```python
from build123d import *

# Parameters (mm, degrees)
BOSS_EXTRUDE1_DEPTH = 5.5
BOSS_EXTRUDE2_DEPTH = 7.5
SKETCH4_R           = 2.5
CUT_EXTRUDE1_DEPTH  = 41.401113846
FILLET1_R           = 2
SKETCH5_R           = 2
FILLET2_RADIUS      = 5.5
FILLET2_LENGTH      = 18
FILLET3_RADIUS      = 5.5
FILLET3_LENGTH      = 18


with BuildPart() as part:
    # Sketch1 → Boss-Extrude1 (new, symmetric)
    with BuildSketch(Plane.XY):
        with BuildLine():
            Line((19, 0), (30, 0))
            Line((30, 0), (30, -18))
            Line((30, -18), (18.761663039, -18))
            ThreePointArc((18.761663039, -18), (0, -26), (-18.761663039, -18))
            Line((-18.761663039, -18), (-30, -18))
            Line((-30, -18), (-30, 0))
            Line((-30, 0), (-19, 0))
            ThreePointArc((-19, 0), (0, -19), (19, 0))
        make_face()
    extrude(amount=BOSS_EXTRUDE1_DEPTH, both=True)

    # Sketch3 → Boss-Extrude2 (add, symmetric)
    with BuildSketch(Plane.XY):
        with BuildLine():
            Line((-21, 0), (-19, 0))
            ThreePointArc((-19, 0), (0, -19), (19, 0))
            Line((19, 0), (21, 0))
            ThreePointArc((21, 0), (0, -21), (-21, 0))
        make_face()
    extrude(amount=BOSS_EXTRUDE2_DEPTH, both=True)

    # Sketch4 → Cut-Extrude1 (cut, through all)
    with BuildSketch(Plane(origin=(0, 0, 0), x_dir=(1, 0, 0), z_dir=(0, 1, 0))):
        with Locations(Location((-24.38083152, 0, 0), (0, 0, 180))):
            Circle(SKETCH4_R)
        with Locations(Location((24.38083152, 0, 0), (0, 0, 180))):
            Circle(SKETCH4_R)
    extrude(amount=-CUT_EXTRUDE1_DEPTH, mode=Mode.SUBTRACT)

    # Fillet1
    fillet1_edges = [part.edges().sort_by_distance(p)[0] for p in [
        (0, -21, -5.5),
        (0, -21, 5.5),
    ]]
    fillet(fillet1_edges, radius=FILLET1_R - 0.0001)  # a hair under: the kernel refuses the full size

    # Sketch5 → Cut-Revolve1 (revolve, cut)
    with BuildSketch(Plane(origin=(0, 0, 0), x_dir=(1, 0, 0), z_dir=(0, 1, 0))):
        with Locations((19, 0)):
            Circle(SKETCH5_R)
    revolve(axis=Axis((0, 0, -5.716287215), (0, 0, 1)), mode=Mode.SUBTRACT)

    # Fillet2: full round fillet: the end face becomes a half cylinder, R = half its width
    fillet2_face = Plane((30, -9, 0), x_dir=(0, 1, 0), z_dir=(1, 0, 0))  # on the end face: x along it, z out of the body
    fillet2_slab = fillet2_face.offset(-FILLET2_RADIUS / 2) * Box(FILLET2_LENGTH, 2 * FILLET2_RADIUS, FILLET2_RADIUS, mode=Mode.PRIVATE)  # the body's end, R deep
    fillet2_round = Plane((24.5, -9, 0), x_dir=(1, 0, 0), z_dir=(0, 1, 0)) * Cylinder(FILLET2_RADIUS, FILLET2_LENGTH, mode=Mode.PRIVATE)  # its axis R under the face
    add(fillet2_slab - fillet2_round, mode=Mode.SUBTRACT)

    # Fillet3: full round fillet: the end face becomes a half cylinder, R = half its width
    fillet3_face = Plane((-30, -9, 0), x_dir=(0, 1, 0), z_dir=(-1, 0, 0))  # on the end face: x along it, z out of the body
    fillet3_slab = fillet3_face.offset(-FILLET3_RADIUS / 2) * Box(FILLET3_LENGTH, 2 * FILLET3_RADIUS, FILLET3_RADIUS, mode=Mode.PRIVATE)  # the body's end, R deep
    fillet3_round = Plane((-24.5, -9, 0), x_dir=(-1, 0, 0), z_dir=(0, 1, 0)) * Cylinder(FILLET3_RADIUS, FILLET3_LENGTH, mode=Mode.PRIVATE)  # its axis R under the face
    add(fillet3_slab - fillet3_round, mode=Mode.SUBTRACT)


solid = part.part
```
The model under review builds one solid part; all positions refer to its coordinate system, in mm. A direction names the side the tool comes from. Round coordinates to 2 decimals unless told otherwise and drop trailing zeros. Order: outer loops, then holes, each group sorted by start corner. A loop starts at its lowest first (then second) coordinate and runs counter-clockwise, first axis right, second up.
(1) For P1, Ø8, axis at y = -20.5, z = 4.5, coming from the -X side; P2, Ø2, axis at x = 4, z = -4, coming from the -Y side; P3, Ø5.5, axis at x = 22.5, z = 0.5, coming from the -Y side, all flat-tipped, find the tip position at first contact; note any pin that passes through.
Working result:
P1: stops at x = -29.82
P2: stops at y = -25.83
P3: stops at y = -18
(2) Mouldability with a two-part tool opening along X and no side actions: class faces 6 (the face through (0, -26, 0)), 7 (the face through (-22, 0, -2)), 8 (the face through (0, -19, -5)) as released by +X, released by -X, zero draft, split by the parting line, or undercut.
Working result:
face 6: split by the parting line
face 7: zero draft
face 8: undercut
(3) Wall thickness on L1, parallel to X at y = -2, z = 2.25; L2, parallel to X at y = -15.75, z = 3.5; L3, parallel to X at y = -15, z = -3.75: over which ranges is each line inside the solid? List them lowest first.
Working result:
L1: x = -29.52 to -25.47, -23.29 to -18.89, 18.89 to 23.29, 25.47 to 29.52
L2: x = -28.74 to -10.63, 10.63 to 28.74
L3: x = -28.52 to -11.66, 11.66 to 28.52
(4) Take a section at D-D, the plane z = 3.75. State the section outline as (x, y) points, plus the area to 3 significant figures.
Working result:
outline: (-28.52, -18) - (-18.76, -18) arc R26 ccw to (18.76, -18) - (28.52, -18) - (28.52, 0) - (19, 0) arc R19 cw to (-19, 0) - (-28.52, 0) - close
area: 667 mm2
(5) Take a section at A-A, the plane z = 0. State the section outline as (x, y) points, plus the area to 3 significant figures.
Working result:
outline: (-30, -18) - (-26.88, -18) - (-26.88, 0) - (-30, 0) - close; (-21.88, -18) - (-18.76, -18) arc R26 ccw to (18.76, -18) - (21.88, -18) - (21.88, 0) - (21, 0) arc R21 cw to (-21, 0) - (-21.88, 0) - close; (26.88, -18) - (30, -18) - (30, 0) - (26.88, 0) - close
area: 415 mm2
(6) Tool access review of faces 1 (the face through (-2, -24, -5.5)), 2 (the face through (-21.8, -18, 1.3)), 3 (the face through (21.96, -18, -1.15)), 4 (the face through (-2, -24, 5.5)), 5 (the face through (-21.883, -8.874, 0.11)): name each direction out of +Z, -Z, +X, -X, +Y, -Y from which nothing blocks a thin tool from reaching the whole face with its end or side.
Working result:
face 1: -Z, -Y
face 2: +Z, -Z, -X, -Y
face 3: +Z, -Z, +X, -Y
face 4: +Z, -Y
face 5: +Y, -Y
(7) Take a section at C-C, the plane y = -5. Count the separate pieces of the cut face and the enclosed holes in it, plus the area to 3 significant figures.
Working result:
separate pieces: 2
enclosed holes: 2
area: 199 mm2
